Build history of the part. All positions in model axes, mm. Face numbers are marked on the shaded views. Round coordinates to 2 decimals unless told otherwise and drop trailing zeros. Write each loop counter-clockwise with the first axis right and the second up, starting at its lowest first coordinate (ties: lowest second). Pieces come first, ordered by that corner, then holes.
Item 1: Band-saw the part on B-B, the plane z = 2.15. Write the cut outline in (x, y).
Item 2: Band-saw the part on D-D, the plane y = 6.5. Write the cut outline in (x, z), then the cut area to 3 significant figures.
Item 3: Band-saw the part on C-C, the plane x = 6.25. Write the cut outline in (y, z), then the cut area to 3 significant figures.
Item 4: Drop a flat-ended pin along its axis: pin 1 Ø3 at (x, z) = (-3, 2) entering from -Y. Give the stop position or say it passes through.
Item 5: Mould opens along X. For the marked faces 1, 2 and 3 say: +X half, -X half, draft (parallel to the pull), parting line (faces both ways), or undercut.
Item 6: Wall check: probe 1 along X at (y, z) = (0, 2.6); probe 2 along X at (y, z) = (-2.5, 3.9); probe 3 along Y at (x, z) = (0.25, 2.85). Give the ranges that are in metal, low to high.
Item 7: Band-saw the part on A-A, the plane y = 0. Write the cut outline in (x, z), then the cut area to 3 significant figures.
Autodesk Inventor part; units mm, degrees
ref_plane "MSC_PT1" through (0, 0, 5) normal (0, 0, 1) x (1, 0, 0)
ref_plane "MSC_PT2" through (0, 0, 0) normal (0, 0, -1) x (-1, 0, 0)
ref_plane "MSC_PF1" through (0, 0, 0) normal (1, 0, 0) x (0, 1, 0)
sketch "Sketch1" plane through (0, 0, 0) normal (0, 0, 1) x (1, 0, 0)
  circle A0 centre (0, 0) radius 8 construction
  line L0 (-8, 4.6188) -> (-8, -4.6188)
  line L1 (-8, -4.6188) -> (0, -9.2376)
  line L2 (0, -9.2376) -> (8, -4.6188)
  line L3 (8, -4.6188) -> (8, 4.6188)
  line L4 (8, 4.6188) -> (0, 9.2376)
  line L5 (0, 9.2376) -> (-8, 4.6188)
  line L6 (0, 12.9326) -> (0, -12.9326)
  line L7 (-11.2, 0) -> (11.2, 0)
  point P0 (0, 0)
  dimension "ParS" = 16
extrude "Extrusion1" add sketch "Sketch1" along normal blind 5
sketch "Sketch2" plane through (0, 0, 5) normal (0, 0, 1) x (1, 0, 0)
  point P0 (0, 0)
  point P1 (0, 0)
hole "Hole1" at (0, 0, 5) direction (0, 0, -1) diameter 8.376 end through all
ref_plane "MSC_PT1" through (0, 0, 5) normal (0, 0, 1) x (1, 0, 0)
ref_plane "MSC_PT2" through (0, 0, 0) normal (0, 0, -1) x (-1, 0, 0)
ref_plane "MSC_PF1" through (0, 0, 0) normal (1, 0, 0) x (0, 1, 0)
chamfer "Chamfer1" distance 0.9 angle 45 2 edges at (0, 4.188, 5) (0, 4.188, 0)
equation "\"d17\" = 0.6 * PTC"
equation "\"d18\" = 0.6 * PTC"
equation "\"d4\" = M"
equation "\"PTC\" = 1.5"
properties part number "ISO 4036 - M10" material "Steel"
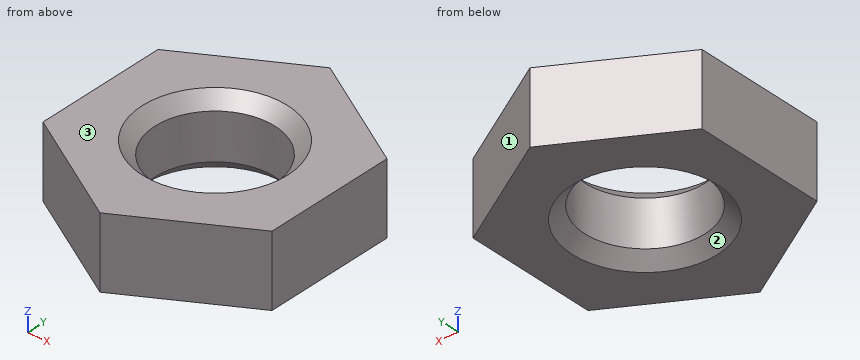
Results:
1. outline: (-8, -4.62) - (0, -9.24) - (8, -4.62) - (8, 4.62) - (0, 9.24) - (-8, 4.62) - close; hole circle Ø8.38 at (0, 0)
2. outline: (-4.74, 0) - (4.74, 0) - (4.74, 5) - (-4.74, 5) - close
2. area: 47.4 mm2
3. outline: (-5.63, 0) - (5.63, 0) - (5.63, 5) - (-5.63, 5) - close
3. area: 56.3 mm2
4. pin 1: stops at y = -8.37
5. face 1: +X half
5. face 2: undercut
5. face 3: draft
6. probe 1: x = -8 to -4.19, 4.19 to 8
6. probe 2: x = -8 to -3.36, 3.36 to 8
6. probe 3: y = -9.09 to -4.18, 4.18 to 9.09
7. outline: (-8, 0) - (-5.09, 0) - (-4.19, 0.9) - (-4.19, 4.1) - (-5.09, 5) - (-8, 5) - close; (4.19, 0.9) - (5.09, 0) - (8, 0) - (8, 5) - (5.09, 5) - (4.19, 4.1) - close
7. area: 36.5 mm2
